Input: dimensioned drawing with shaded views. Units: mm. Origin: part minimum x, y, z. Coordinates: 2 decimals unless noted, no trailing zeros. Loops run counter-clockwise (first coordinate to the right, second up) from the corner with the lowest first, then second, coordinate; pieces in that order, holes last. Notation, with made-up numbers: (-11, 17.5) - (-3, 17.5) arc R32 ccw to (-3, 45.5) - close; hole circle Ø4 at (-21.75, 89). An arc over 180 degrees is marked (long way). Write item = value, one per line. Start each with the question number.
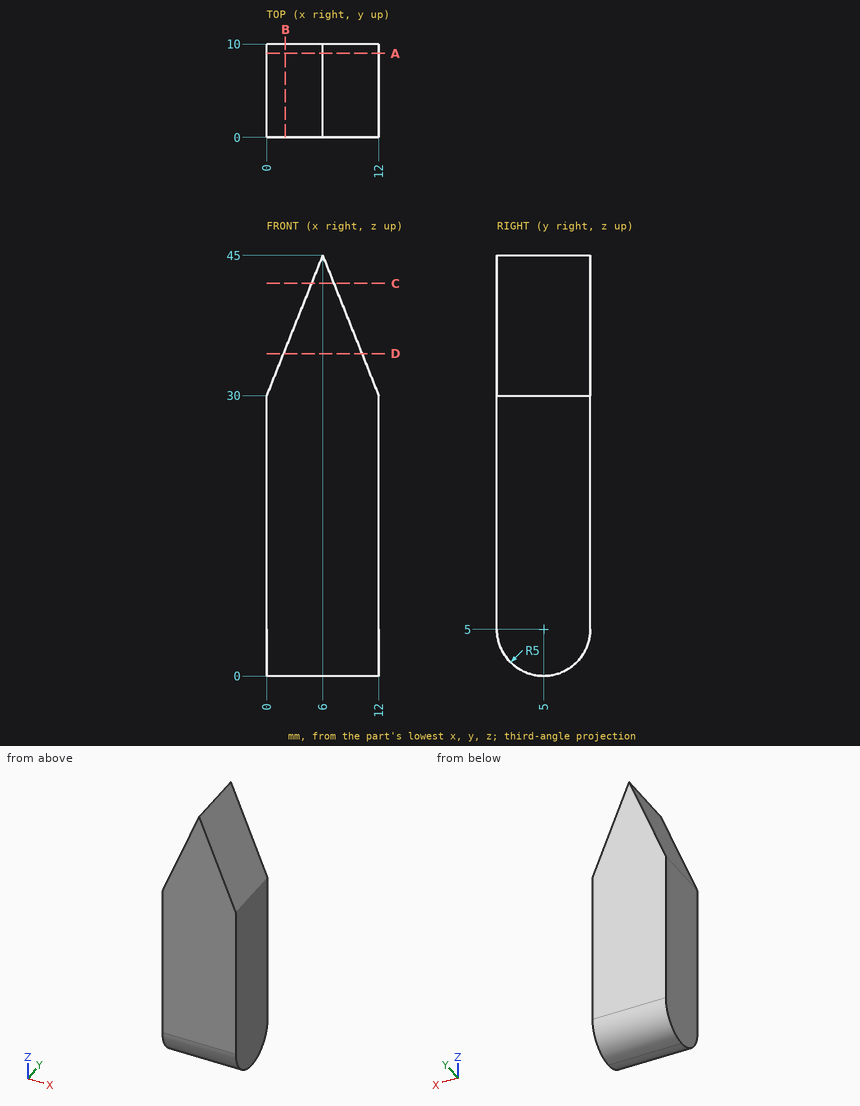
Item 1: Cut plane A-A on y = 9. Return loops of the section in (x, z), plus the area to 3 significant figures.
Item 2: Ray query, line 1 (X direction, y = 6, z = 43); line 2 (X direction, y = 8.5, z = 32.5); line 3 (Y direction, x = 7.5, z = 4). Return the intervals inside material, ascending.
Item 3: Cut plane C-C on z = 42. Return loops of the section in (x, y).
Item 4: Cut plane D-D on z = 34.5. Return loops of the section in (x, y), plus the area to 3 significant figures.
Item 5: Cut plane B-B on x = 2. Return loops of the section in (y, z).
Item 6: Pin query (flat end, axial travel): pin 1 (6 mm diameter, centred on x = 8.5, y = 1.5, fed in from -Z). Return the tip coordinate at first contact, or that it passes through.
Recorded:
q1.outline = (0, 2) - (12, 2) - (12, 30) - (6, 45) - (0, 30) - close
q1.area = 426 mm²
q2.line_1 = 5.2 to 6.8
q2.line_2 = 1 to 11
q2.line_3 = 0.1 to 9.9
q3.outline = (4.8, 0) - (7.2, 0) - (7.2, 10) - (4.8, 10) - close
q4.outline = (1.8, 0) - (10.2, 0) - (10.2, 10) - (1.8, 10) - close
q4.area = 84.0 mm²
q5.outline = (0, 5) arc R5 ccw to (10, 5) - (10, 35) - (0, 35) - close
q6.pin_1 = 0.03
